Part model, mm, in its own coordinate system. A direction names the side the tool comes from. Give positions to 0.01 mm unless a question says otherwise; leave off trailing zeros. Loops run counter-clockwise (first coordinate to the right, second up) from the corner with the lowest first, then second, coordinate; pieces in that order, holes last. Notation, with made-up numbers: (-12.75, 50.5) -> (40.25, 50.5) arc R36 ccw to (40.25, 85.5) -> close; hole circle Ø1 at (79.25, -17). An arc over 180 degrees is marked (long way). Write item = value, one per line.
Solid Edge part; units mm, degrees
sketch "Sketch1" plane through (0, 0, 0) normal (0, 0, 1) x (1, 0, 0)
  circle A0 centre (0, 0) radius 4
extrude "Ajout_matière_1" add sketch "Sketch1" along normal blind 404
chamfer "Chanfrein_1" distance 1 angle 45 2 edges at (-4, 0, 404) (-4, 0, 0)
sketch "Sketch2" plane through (0, 0, 0) normal (0, -1, 0) x (1, 0, 0)
  line L0 (3, 5) -> (3, 6.5)
  line L1 (3, 6.5) -> (4, 6.5)
  line L2 (4, 6.5) -> (5.3414, 6.5)
  line L3 (5.3414, 6.5) -> (5.3414, 5)
  line L4 (3, 5) -> (5.3414, 5)
  line L5 (3, 397.5) -> (6.5, 397.5)
  line L6 (6.5, 397.5) -> (6.5, 399)
  line L7 (6.5, 399) -> (3, 399)
  line L8 (3, 399) -> (3, 397.5)
  dimension "D1" = 3
  dimension "D2" = 3
  dimension "D3" = 3
  dimension "D4" = 3
revolve "RevolvedCutout1" cut sketch "Sketch2" angle 360 about axis through (0, 0, 54) along (0, 0, -1)
properties material "Acier S235"
1) Slice it at A-A, the plane z = 119.5. List the corners of the cut face in (x, y).
Resolved:
outline = circle Ø8 at (0, 0)
2) Pull direction Z, two halves, no side cores. Call faces 3 (the face through (-0.867, 3.905, 199.263)), 4 (the face through (1, -3, 6.5)): pulls with the +Z half, pulls with the -Z half, needs draft (parallel to the pull), parting line crosses it, or undercut.
Resolved:
face_3 = needs draft
face_4 = undercut
3) Which spindle directions (+Z, -Z, +X, -X, +Y, -Y) get a long thin tool onto all of the face, cutting with end or side? Do faces 1 (the face through (1, -3, 397.5)), 2 (the face through (-0.867, 3.905, 400.972)). Say none if no direction does.
Resolved:
face_1 = none
face_2 = +Z, -Z
4) Drill centre lines: line 1 along Z through (x, y) = (-3, 2.25); line 2 along Z through (x, y) = (3, 2); line 3 along Y through (x, z) = (0.25, 143.5). Where is each one in solid material? Low to high. Write a range as [from, to].
Resolved:
line_1 = [0.75, 5], [6.5, 397.5], [399, 403.25]
line_2 = [0.61, 5], [6.5, 397.5], [399, 403.39]
line_3 = [-3.99, 3.99]
5) Drop a flat-ended pin along its axis: P1, Ø1, axis at y = -2.5, z = 141, coming from the -X side. Give the stop position or say it passes through.
Resolved:
P1 = -3.46
